from build123d import *

# Parameters (mm, degrees)
BOSS_EXTRUDE1_DEPTH = 1250
SKETCH4_R           = 22.750036828
CUT_EXTRUDE1_DEPTH  = 361.95


with BuildPart() as part:
    # Sketch3 → Boss-Extrude1 (new, symmetric)
    with BuildSketch(Plane.XY):
        with BuildLine():
            Line((6.350000091, 12.7), (9.5758, 12.7))
            ThreePointArc((9.5758, 12.7), (10.0838, 12.192), (10.5918, 12.7))
            ThreePointArc((10.5918, 12.7), (11.398573212, 12.53952283), (12.082522516, 12.082522516))
            Line((12.082522516, 12.082522516), (1.841111635, 1.841111635))
            ThreePointArc((1.841111635, 1.841111635), (-1.841111635, 1.841111635), (-1.841111635, -1.841111635))
            Line((-1.841111635, -1.841111635), (-3.170518398, -3.170518398))
            ThreePointArc((-3.170518398, -3.170518398), (-4.284365606, -1.322340795), (-4.405901938, 0.832106923))
            ThreePointArc((-4.405901938, 0.832106923), (-4.49196258, 2.357684911), (-5.280684798, 3.666391103))
            Line((-5.280684798, 3.666391103), (-8.603375093, 6.989081397))
            ThreePointArc((-8.603375093, 6.989081397), (-9.812092525, 7.226672612), (-10.489512256, 6.197814058))
            ThreePointArc((-10.489512256, 6.197814058), (-9.179037358, -0.164701156), (-5.55781952, -5.55781952))
            Line((-5.55781952, -5.55781952), (-7.120384159, -7.120384159))
            ThreePointArc((-7.120384159, -7.120384159), (-8.636327096, -5.410633429), (-9.936651338, -3.531674301))
            ThreePointArc((-9.936651338, -3.531674301), (-9.753165795, -2.842051688), (-10.440280632, -2.649387487))
            ThreePointArc((-10.440280632, -2.649387487), (-11.049200851, -1.406952263), (-11.566334617, -0.123596589))
            ThreePointArc((-11.566334617, -0.123596589), (-11.250376175, 0.51626008), (-11.885963187, 0.840721857))
            ThreePointArc((-11.885963187, 0.840721857), (-12.495391993, 3.565453333), (-12.7, 6.350000091))
            Line((-12.7, 6.350000091), (-12.7, 9.5758))
            ThreePointArc((-12.7, 9.5758), (-12.192, 10.0838), (-12.7, 10.5918))
            ThreePointArc((-12.7, 10.5918), (-12.082522516, 12.082522516), (-10.5918, 12.7))
            ThreePointArc((-10.5918, 12.7), (-10.0838, 12.192), (-9.5758, 12.7))
            Line((-9.5758, 12.7), (-6.350000091, 12.7))
            ThreePointArc((-6.350000091, 12.7), (-5.842000091, 12.192), (-5.334000091, 12.7))
            Line((-5.334000091, 12.7), (-4.3561, 12.7))
            ThreePointArc((-4.3561, 12.7), (-3.2512, 11.5951), (-4.3561, 10.4902))
            Line((-4.3561, 10.4902), (-6.3119, 10.4902))
            ThreePointArc((-6.3119, 10.4902), (-7.332694495, 9.808126924), (-7.093182283, 8.604017717))
            Line((-7.093182283, 8.604017717), (-3.914900535, 5.42573597))
            ThreePointArc((-3.914900535, 5.42573597), (-2.884856402, 4.737482484), (-1.669836505, 4.4958))
            Line((-1.669836505, 4.4958), (1.669836505, 4.4958))
            ThreePointArc((1.669836505, 4.4958), (2.884856402, 4.737482484), (3.914900535, 5.42573597))
            Line((3.914900535, 5.42573597), (7.093182283, 8.604017717))
            ThreePointArc((7.093182283, 8.604017717), (7.332694495, 9.808126924), (6.3119, 10.4902))
            Line((6.3119, 10.4902), (4.3561, 10.4902))
            ThreePointArc((4.3561, 10.4902), (3.2512, 11.5951), (4.3561, 12.7))
            Line((4.3561, 12.7), (5.334000091, 12.7))
            ThreePointArc((5.334000091, 12.7), (5.842000091, 12.192), (6.350000091, 12.7))
        make_face()
    extrude(amount=BOSS_EXTRUDE1_DEPTH, both=True)

    # Mirror1: part across plane


with BuildPart() as part_1:
    add(part.part)
    add(part.part.mirror(Plane(origin=(1.841111635, 1.841111635, 1250), x_dir=(0, 0, 1), z_dir=(-0.707106781186552, 0.707106781186543, 0))))

    # Sketch4 → Cut-Extrude1 (cut)
    with BuildSketch(Plane.XY.offset(1250)):
        Circle(SKETCH4_R)
    extrude(amount=-CUT_EXTRUDE1_DEPTH, mode=Mode.SUBTRACT)


solid = part_1.part
Can you work these out from the model? Positions are in its coordinate system, mm. Round coordinates to 2 decimals unless told otherwise and drop trailing zeros. One line per question, with ' | ' between items. Start each with the question number.
1) Suppose I cut it at A-A on z = -925. Count the separate pieces of the cut face and the enclosed holes in it, then the cut area to 3 significant figures.
2) I'm going to push flat-ended pins straight in: P1, Ø0.6, axis at x = -5, z = -346.5, coming from the -Y side; P2, Ø3.5, axis at y = 1, z = -507, coming from the +X side; P3, Ø3, axis at y = -6, z = 255.5, coming from the -X side. Where does each tip first touch, or does it pass through?
3) I need wall thicknesses on line 1 (Y direction, x = 0, z = -547.5); line 2 (Y direction, x = -3.75, z = -1117). Which ranges of each line are inside material? Lowest first, please. Write a range as [from, to].
Return value:
1) separate pieces: 1 | enclosed holes: 2 | area: 269 mm2
2) P1: stops at y = -9.17 | P2: stops at x = 4.69 | P3: stops at x = -9.31
3) line 1: y = [-11.37, -9.25], [-4.48, -2.6], [2.6, 4.5] | line 2: y = [-9.8, -7.13], [-2.46, 5.27], [10.67, 12.52]
